Autodesk Inventor part; units mm, degrees
ref_plane "YZ Plane" through (0, 0, 0) normal (1, 0, 0) x (0, 1, 0)
ref_plane "XZ Plane" through (0, 0, 0) normal (0, 1, 0) x (-1, 0, 0)
ref_plane "XY Plane" through (0, 0, 0) normal (0, 0, 1) x (1, 0, 0)
sketch "Sketch1" plane through (0, 0, 0) normal (0, 0, 1) x (1, 0, 0)
  circle A0 centre (0, 0) radius 2.1844
  circle A1 centre (25.4, 0) radius 2.1844
  circle A2 centre (50.8, 0) radius 2.1844
  line L0 (0, 6.35) -> (50.8, 6.35)
  line L1 (0, -6.35) -> (50.8, -6.35)
  arc A3 (0, 6.35) -> (0, -6.35) centre (0, 0) ccw
  arc A4 (50.8, -6.35) -> (50.8, 6.35) centre (50.8, 0) ccw
  dimension "d0" = 4.3688
  dimension "d1" = 4.3688
  dimension "d2" = 25.4
  dimension "d3" = 4.3688
  dimension "d4" = 25.4
extrude "Extrusion1" add sketch "Sketch1" along normal blind 1.5875
properties part number "gearbox bracket"
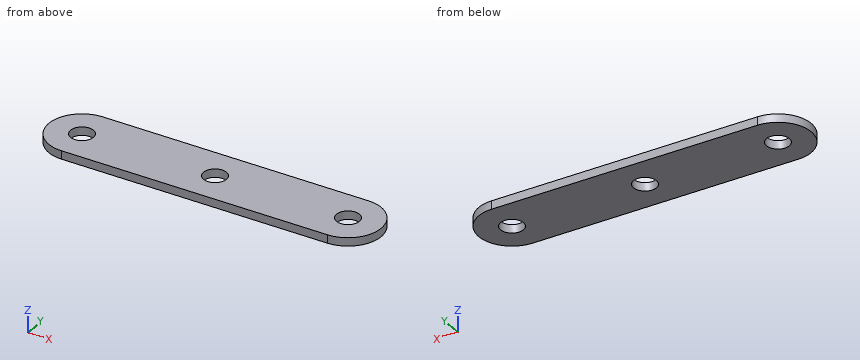
Read the model definition and answer for the solid it produces. Units are mm, in the model's axes. Give positions to 0.01 mm unless a question says otherwise; leave off trailing zeros. Write each loop counter-clockwise with the first axis right and the second up, starting at its lowest first coordinate (ties: lowest second). Pieces come first, ordered by that corner, then holes. Notation, with made-up numbers: (58, 57) - (85, 57) arc R21 cw to (85, 71) - close; hole circle Ø6 at (48, 46.5). An arc over 180 degrees is marked (long way). Return JSON: item names as keys, results as strings.
Q1. Consider line 1 along Y through (x, z) = (25.4, 0.8); line 2 along X through (y, z) = (0.25, 0.55). Determine where each line is inside the solid, lowest interval first. Write a range as [from, to].
Reply:
{"line 1": "[-6.35, -2.18], [2.18, 6.35]", "line 2": "[-6.35, -2.17], [2.17, 23.23], [27.57, 48.63], [52.97, 57.15]"}
Q2. A cutting plane is placed at C-C, the plane y = -1. Determine the outline of the cut face in (x, z), and give its area (3 significant figures).
Reply:
{"outline": "(-6.27, 0) - (-1.94, 0) - (-1.94, 1.59) - (-6.27, 1.59) - close; (1.94, 0) - (23.46, 0) - (23.46, 1.59) - (1.94, 1.59) - close; (27.34, 0) - (48.86, 0) - (48.86, 1.59) - (27.34, 1.59) - close; (52.74, 0) - (57.07, 0) - (57.07, 1.59) - (52.74, 1.59) - close", "area": "82.1 mm²"}
Q3. A cutting plane is placed at B-B, the plane x = 25.4. Determine the outline of the cut face in (y, z), and give its area (3 significant figures).
Reply:
{"outline": "(-6.35, 0) - (-2.18, 0) - (-2.18, 1.59) - (-6.35, 1.59) - close; (2.18, 0) - (6.35, 0) - (6.35, 1.59) - (2.18, 1.59) - close", "area": "13.2 mm²"}
Q4. A cutting plane is placed at A-A, the plane z = 1.05. Determine the outline of the cut face in (x, y).
Reply:
{"outline": "(0, -6.35) - (50.8, -6.35) arc R6.35 ccw to (50.8, 6.35) - (0, 6.35) arc R6.35 ccw to start; hole circle Ø4.37 at (0, 0); hole circle Ø4.37 at (25.4, 0); hole circle Ø4.37 at (50.8, 0)"}
Q5. A cutting plane is placed at D-D, the plane y = -4. Determine the outline of the cut face in (x, z).
Reply:
{"outline": "(-4.93, 0) - (55.73, 0) - (55.73, 1.59) - (-4.93, 1.59) - close"}
Q6. Given P1, Ø4, axis at x = 50.8, y = 0, coming from the -Z side; P2, Ø5.5, axis at x = 25.4, y = 0, coming from the +Z side, each flat-ended and moving along its own axis, determine where each tip first touches the part or whether it passes through.
Reply:
{"P1": "through", "P2": "z = 1.59"}
